Check sheet for the modelled part. Datum: model origin and axes. Units: mm. A direction names the side the tool comes from. Give positions to 0.01 mm unless a question says otherwise; leave off trailing zeros. Order: outer loops, then holes, each group sorted by start corner. A loop starts at its lowest first (then second) coordinate and runs counter-clockwise, first axis right, second up. Notation, with made-up numbers: (-5, -16) -> (-1, -16) arc R32 ccw to (-1, 18) -> close; hole circle Ø5 at (-39.75, 38.25). An arc over 180 degrees is marked (long way). Answer in a Markdown table with one row per item. Add a question column.
(1) Release check for a two-part mould opening along X. For faces 4 (the face through (73.427, 2.103, 15.563)), 5 (the face through (-13.17, -98.1, 17.22)), 6 (the face through (-44, 5, 40)), 7 (the face through (-1.63, -115.31, 13.88)) record: released by +X, released by -X, zero draft, split by the parting line, or undercut.
(2) Go/stop test with flat-tipped pins: pin 1 (6 mm diameter, centred on x = 38, y = 22.5, fed in from +Z); pin 2 (10 mm diameter, centred on y = -2.5, z = 32, fed in from +X); pin 3 (19 mm diameter, centred on x = 8.5, z = 47, fed in from -Y); pin 4 (7 mm diameter, centred on x = 66.75, y = 0, fed in from +Z) (3 decimals). Record where each tip stops, or that it passes through.
(3) Cross-section at B-B (z = 62.5). Record the cut outline in (x, y).
(4) Thickness scan on L1, parallel to Y at x = 66, z = 17; L2, parallel to Y at x = 3, z = 24; L3, parallel to Z at x = 0, y = -96. Record the ranges inside material, lowest first. Write a range as [from, to].
(5) Cross-section at C-C (x = 66.75). Record the cut outline in (y, z), then the cut area to 3 significant figures.
(6) Cross-section at A-A (y = -23.5). Record the cut outline in (x, z), then the cut area to 3 significant figures.
(7) Set-up check for faces 1 (the face through (37, -65.5, 30)), 2 (the face through (-1, 1, 20)), 3 (the face through (-72.305, -4.259, 15.563)): record each of +Z, -Z, +X, -X, +Y, -Y from which the full face is reachable in a straight line by a thin tool's end or side.
(8) Cross-section at D-D (y = 40). State how many separate pieces and enclosed holes the cut face has, then the cut area to 3 significant figures.
```python
from build123d import *

# Parameters (mm, degrees)
F0_W         = 164
F0_H         = 170
F0_R         = 4.25
F0_R_2       = 5
F1_DEPTH     = 20
F3_SIZE      = 2
F4_DEPTH     = 20
F2_R         = 7
F2_R_2       = 4.25
F5_DEPTH     = 9
F6_W         = 20
F6_H         = 140
F7_DEPTH     = 20
F8_W         = 5.5
F8_H         = 140
F9_DEPTH     = 5
F10_W        = 38.5
F10_H        = 2.8
F10_H_2      = 11.2
F11_DEPTH    = 67.5
F12_W        = 38.5
F12_H        = 14
F13_DEPTH    = 179
F14_W        = 38.5
F14_H        = 14
F15_DEPTH    = 62.2
F16_SIZE     = 12
F17_R        = 4.5
F18_DEPTH    = 14
F19_R        = 7.5
F19_R_2      = 4.5
F20_DEPTH    = 19
F21_R        = 11
F21_R_2      = 7.5
F22_DEPTH    = 11
F23_S5_R     = 7.5
F23_T6_DEPTH = 17
F24_R        = 2
F25_W        = 38.5
F25_H        = 16
F25_H_2      = 5
F26_DEPTH    = 15.5
F27_SIZE2    = 5
F27_SIZE     = 10


# Not quite as in the source:
# - a fillet or chamfer that OpenCascade refuses, or shapes differently, is made with other operations: its cross-section is extruded or revolved along the edge and cut away or added


with BuildPart() as f1:
    # F0 (on Top) → F1 (new body)
    with BuildSketch(Plane.XY):
        Rectangle(F0_W, F0_H)
        with Locations((-66.75, 0)):
            Circle(F0_R, mode=Mode.SUBTRACT)
        with Locations((0, 40)):
            Circle(F0_R_2, mode=Mode.SUBTRACT)
        with Locations((66.75, 0)):
            Circle(F0_R, mode=Mode.SUBTRACT)
    extrude(amount=F1_DEPTH)

    # F3
    f3_edges = [f1.edges().sort_by_distance(p)[0] for p in [
        (82, 0, 20),
        (0, -85, 20),
        (0, 85, 20),
        (-82, 0, 20),
    ]]
    chamfer(f3_edges, length=F3_SIZE)

    # F0 (on Top) → F4 (cut)
    with BuildSketch(Plane.XY):
        with Locations((0, 40)):
            Circle(F0_R_2)
    extrude(amount=F4_DEPTH, mode=Mode.SUBTRACT)

    # F2 (on face) → F5 (cut)
    with BuildSketch(Plane.XY.offset(20)):
        with Locations((-66.75, 0)):
            Circle(F2_R)
        with Locations((-66.75, 0)):
            Circle(F2_R_2, mode=Mode.SUBTRACT)
        with Locations((66.75, 0)):
            Circle(F2_R)
        with Locations((66.75, 0)):
            Circle(F2_R_2, mode=Mode.SUBTRACT)
    extrude(amount=-F5_DEPTH, mode=Mode.SUBTRACT)

    # F6 (on face) → F7 (join)
    with BuildSketch(Plane.XY.offset(20)):
        with Locations((-37.5, 4.5)):
            Rectangle(F6_W, F6_H)
        with Locations((37.5, 4.5)):
            Rectangle(F6_W, F6_H)
    extrude(amount=F7_DEPTH)

    # F8 (on face) → F9 (cut)
    with BuildSketch(Plane.XY.offset(40)):
        with Locations((-37.5, 4.5)):
            Rectangle(F8_W, F8_H)
        with Locations((37.5, 4.5)):
            Rectangle(F8_W, F8_H)
    extrude(amount=-F9_DEPTH, mode=Mode.SUBTRACT)

    # F10 (on face) → F11 (join)
    with BuildSketch(Plane.XY.offset(20)):
        with Locations((0, 86.4)):
            Rectangle(F10_W, F10_H)
        with Locations((0, 79.4)):
            Rectangle(F10_W, F10_H_2)
    extrude(amount=F11_DEPTH)

    # F12 (on face) → F13 (join)
    with BuildSketch(Plane.XZ.offset(-73.8)):
        with Locations((0, 80.5)):
            Rectangle(F12_W, F12_H)
    extrude(amount=F13_DEPTH)

    # F14 (on face) → F15 (join)
    with BuildSketch(Plane(origin=(0, 0, 73.5), x_dir=(1, 0, 0), z_dir=(0, 0, -1))):
        with Locations((0, 98.2)):
            Rectangle(F14_W, F14_H)
    extrude(amount=F15_DEPTH)

    # F16
    f16_edges = [f1.edges().sort_by_distance(p)[0] for p in [
        (-19.25, -98.2, 11.3),
        (19.25, -98.2, 11.3),
    ]]
    chamfer(f16_edges, length=F16_SIZE)

    # F17 (on face) → F18 (cut)
    with BuildSketch(Plane.XZ.offset(105.2)):
        with Locations((0, 21.2)):
            Circle(F17_R)
    extrude(amount=-F18_DEPTH, mode=Mode.SUBTRACT)

    # F19 (on face) → F20 (join)
    with BuildSketch(Plane.XZ.offset(105.2)):
        with Locations((0, 21.2)):
            Circle(F19_R)
        with Locations((0, 21.2)):
            Circle(F19_R_2, mode=Mode.SUBTRACT)
        with Locations((0, 21.2)):
            Circle(F19_R_2)
    extrude(amount=F20_DEPTH)

    # F21 (on face) → F22 (join)
    with BuildSketch(Plane.XZ.offset(124.2)):
        with Locations((0, 21.2)):
            Circle(F21_R)
        with Locations((0, 21.2)):
            Circle(F21_R_2, mode=Mode.SUBTRACT)
        with Locations((0, 21.2)):
            Circle(F21_R_2)
    extrude(amount=F22_DEPTH)

    # F23: chamfer of 5 on 1 edges, made by hand


with BuildPart() as f23_tool2:
    # F23_s3 → F23_t4 (revolve)
    with BuildSketch(Plane.XY.offset(21.2)):
        Polygon((11, -129.2), (6, -124.2), (11, -124.2), align=None)
    revolve(axis=Axis((0, -124.2, 21.2), (0, -1, 0)))

    # F23_s5 → F23_t6 (cut, symmetric)
    with BuildSketch(Plane.XZ.offset(126.7)):
        with Locations((0, 21.2)):
            Circle(F23_S5_R)
    extrude(amount=F23_T6_DEPTH, both=True, mode=Mode.SUBTRACT)


with BuildPart() as f1_1:
    add(f1.part)

    # F23_t1: cut F23_tool2
    add(f23_tool2.part, mode=Mode.SUBTRACT)

    # F24
    f24_edges = [f1_1.edges().sort_by_distance(p)[0] for p in [
        (-11, -135.2, 21.2),
    ]]
    fillet(f24_edges, radius=F24_R)

    # F25 (on face) → F26 (join)
    with BuildSketch(Plane.XY.offset(20)):
        with Locations((0, -77)):
            Rectangle(F25_W, F25_H)
        with Locations((0, -87.5)):
            Rectangle(F25_W, F25_H_2)
    extrude(amount=F26_DEPTH)

    # F27
    f27_edges = [f1_1.edges().sort_by_distance(p)[0] for p in [
        (0, -90, 35.5),
    ]]
    f27_side = f1_1.faces().sort_by_distance((0, -90, 27.75))[0]
    chamfer(f27_edges, length=F27_SIZE, length2=F27_SIZE2, reference=f27_side)


solid = f1_1.part
```
Answer below:
| question | item | result |
|---|---|---|
| 1 | face 4 | undercut |
| 1 | face 5 | released by -X |
| 1 | face 6 | zero draft |
| 1 | face 7 | split by the parting line |
| 2 | pin 1 | stops at z = 40 |
| 2 | pin 2 | stops at x = 47.5 |
| 2 | pin 3 | stops at y = -105.2 |
| 2 | pin 4 | passes through |
| 3 | outline | (-19.25, -105.2) -> (19.25, -105.2) -> (19.25, -91.2) -> (-19.25, -91.2) -> close; (-19.25, 73.8) -> (19.25, 73.8) -> (19.25, 87.8) -> (-19.25, 87.8) -> close |
| 4 | L1 | y = [-85, -6.96], [6.96, 85] |
| 4 | L2 | y = [-135.2, -105.2], [-90, -69], [73.8, 87.8] |
| 4 | L3 | z = [11.3, 16.7], [25.7, 87.5] |
| 5 | outline | (-85, 0) -> (-4.25, 0) -> (-4.25, 11) -> (-7, 11) -> (-7, 20) -> (-83, 20) -> (-85, 18) -> close; (4.25, 0) -> (85, 0) -> (85, 18) -> (83, 20) -> (7, 20) -> (7, 11) -> (4.25, 11) -> close |
| 5 | area | 3,180 mm² |
| 6 | outline | (-82, 0) -> (82, 0) -> (82, 18) -> (80, 20) -> (47.5, 20) -> (47.5, 40) -> (40.25, 40) -> (40.25, 35) -> (34.75, 35) -> (34.75, 40) -> (27.5, 40) -> (27.5, 20) -> (-27.5, 20) -> (-27.5, 40) -> (-34.75, 40) -> (-34.75, 35) -> (-40.25, 35) -> (-40.25, 40) -> (-47.5, 40) -> (-47.5, 20) -> (-80, 20) -> (-82, 18) -> close; (-19.25, 73.5) -> (19.25, 73.5) -> (19.25, 87.5) -> (-19.25, 87.5) -> close |
| 6 | area | 4,560 mm² |
| 7 | face 1 | +Z, +X, -X, -Y |
| 7 | face 2 | none |
| 7 | face 3 | +Z |
| 8 | separate pieces | 3 |
| 8 | enclosed holes | 0 |
| 8 | area | 4,360 mm² |
